Geometry check sheet. Reference: the model listing, model coordinates, mm. Round coordinates to 2 decimals unless told otherwise and drop trailing zeros. Order: outer loops, then holes, each group sorted by start corner. A loop starts at its lowest first (then second) coordinate and runs counter-clockwise, first axis right, second up. Notation, with made-up numbers: (-14, -24) - (2, -24) arc R33 cw to (2, 13) - close; hole circle Ø11 at (36, -6). An arc over 180 degrees is marked (long way). One line per question, with ' | ' between items. Start each with the question number.
Q1. Sectioned sample at B-B, the plane x = 251. Enter the section's corners in (y, z).
Q2. Material ranges on line 1 along X through (y, z) = (2.6, -21.25) (3 decimals); line 2 along X through (y, z) = (3.1, -8.5) (3 decimals); line 3 along X through (y, z) = (1.2, -90), recorded low to high.
Q3. Sectioned sample at A-A, the plane y = 1.65. Give the number of separate pieces and of enclosed holes in the cut face, then the cut area to 3 significant figures.
Q4. Gauge pin test, flat ends, axial feed: P1, Ø1.2, axis at x = 226, y = 1, coming from the +Z side; P2, Ø1, axis at x = 83.5, z = -84.5, coming from the -Y side; P3, Ø2, axis at x = 2, y = 2.5, coming from the -Z side; P4, Ø2, axis at x = 498, y = 1.5, coming from the +Z side. Record the tip position at first contact, or that the pin passes through.
```python
from build123d import *

# Parameters (mm, degrees)
SKETCH1_R           = 2.125
SKETCH1_W           = 19.725
SKETCH1_H           = 4
BOSS_EXTRUDE1_DEPTH = 4


with BuildPart() as part:
    # Sketch1 → Boss-Extrude1 (new body)
    with BuildSketch(Plane(origin=(0, 0, 0), x_dir=(1, 0, 0), z_dir=(0, 1, 0))):
        Polygon((4, 0), (4, 20), (0, 20), (0, 40), (4, 40), (4, 60), (0, 60), (0, 80), (4, 80), (4, 100), (250, 100), (496, 100), (496, 80), (500, 80), (500, 60), (496, 60), (496, 40), (500, 40), (500, 20), (496, 20), (496, 0), (476, 0), (476, 70), (24, 70), (24, 0), align=None)
        with Locations((14, 8.5)):
            Circle(SKETCH1_R, mode=Mode.SUBTRACT)
        with Locations((14, 21.25)):
            Circle(SKETCH1_R, mode=Mode.SUBTRACT)
        with Locations((173.885, 90)):
            Circle(SKETCH1_R, mode=Mode.SUBTRACT)
        with Locations((326.115, 90)):
            Circle(SKETCH1_R, mode=Mode.SUBTRACT)
        with Locations((486, 21.25)):
            Circle(SKETCH1_R, mode=Mode.SUBTRACT)
        with Locations((486, 8.5)):
            Circle(SKETCH1_R, mode=Mode.SUBTRACT)
        with Locations((63.3125, 78)):
            Rectangle(SKETCH1_W, SKETCH1_H, mode=Mode.SUBTRACT)
        with Locations((23.8625, 78)):
            Rectangle(SKETCH1_W, SKETCH1_H, mode=Mode.SUBTRACT)
        with Locations((102.7625, 78)):
            Rectangle(SKETCH1_W, SKETCH1_H, mode=Mode.SUBTRACT)
        with Locations((142.2125, 78)):
            Rectangle(SKETCH1_W, SKETCH1_H, mode=Mode.SUBTRACT)
        with Locations((181.6625, 78)):
            Rectangle(SKETCH1_W, SKETCH1_H, mode=Mode.SUBTRACT)
        with Locations((221.1125, 78)):
            Rectangle(SKETCH1_W, SKETCH1_H, mode=Mode.SUBTRACT)
        with Locations((278.8875, 78)):
            Rectangle(SKETCH1_W, SKETCH1_H, mode=Mode.SUBTRACT)
        with Locations((318.3375, 78)):
            Rectangle(SKETCH1_W, SKETCH1_H, mode=Mode.SUBTRACT)
        with Locations((357.7875, 78)):
            Rectangle(SKETCH1_W, SKETCH1_H, mode=Mode.SUBTRACT)
        with Locations((397.2375, 78)):
            Rectangle(SKETCH1_W, SKETCH1_H, mode=Mode.SUBTRACT)
        with Locations((436.6875, 78)):
            Rectangle(SKETCH1_W, SKETCH1_H, mode=Mode.SUBTRACT)
        with Locations((476.1375, 78)):
            Rectangle(SKETCH1_W, SKETCH1_H, mode=Mode.SUBTRACT)
    extrude(amount=BOSS_EXTRUDE1_DEPTH)


solid = part.part
```
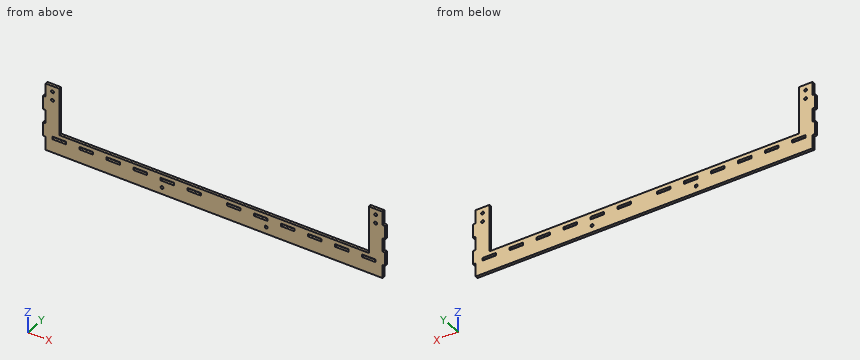
Determined:
1) outline: (0, -100) - (4, -100) - (4, -70) - (0, -70) - close
2) line 1: x = 0 to 11.875, 16.125 to 24, 476 to 483.875, 488.125 to 500 | line 2: x = 4 to 11.875, 16.125 to 24, 476 to 483.875, 488.125 to 496 | line 3: x = 4 to 171.76, 176.01 to 323.99, 328.24 to 496
3) separate pieces: 1 | enclosed holes: 18 | area: 16,800 mm2
4) P1: stops at z = -70 | P2: stops at y = 0 | P3: stops at z = -80 | P4: stops at z = -20
